Design review of the part built by this model. Coordinates are the model's own, in mm. Give positions to 0.01 mm unless a question says otherwise; leave off trailing zeros. Loops run counter-clockwise (first coordinate to the right, second up) from the corner with the lowest first, then second, coordinate; pieces in that order, holes last. Notation, with made-up numbers: M -14,1.25 L 21,1.25 A15 cw 21,15.25 Z; hole C 8.25,9 d4. An arc over 180 degrees is marked long. Use a Markdown table: item, result. Add a question column.
(1) Add section A-A, the plane y = 5. Give the boundary of the cut face in (x, z).
(2) For probe 1 along X at (y, z) = (5.5, 0.4); probe 2 along X at (y, z) = (2.75, 1.05); probe 3 along Y at (x, z) = (1.5, 0.6), list the stretches that pass through material, from the lowest coordinate up.
(3) Add section C-C, the plane z = 0.5. State how many separate pieces and enclosed holes the cut face has, then the cut area to 3 significant figures.
(4) Draft analysis for pull direction X (two halves, no side actions). For faces 1 (the face through (-2.356, 5, 1)), 2 (the face through (14.89, 3.13, 0.74)), 3 (the face through (9, 5, 0)), state which applies: pulls with the +X half, pulls with the -X half, needs draft (parallel to the pull), parting line crosses it, or undercut.
(5) Insertion check: pin 1 Ø3 at (x, y) = (16.64, 4.73) entering from +Z. The pin has a flat end and moves straight along its axis. Give the tip position at first contact, or say it passes through.
(6) Add section B-B, the plane x = 15.5. Give the boundary of the cut face in (y, z).
Autodesk Inventor part; units mm, degrees
ref_plane "YZ Plane" through (0, 0, 0) normal (1, 0, 0) x (0, 1, 0)
ref_plane "XZ Plane" through (0, 0, 0) normal (0, 1, 0) x (-1, 0, 0)
ref_plane "XY Plane" through (0, 0, 0) normal (0, 0, 1) x (1, 0, 0)
sketch "Sketch2" plane through (0, 0, 0) normal (0, 0, 1) x (1, 0, 0)
  circle A0 centre (1.6435, 4.7319) radius 2.125
  circle A1 centre (1.6435, 4.7319) radius 2.375
  line L0 (1.6435, 4.7319) -> (1.6435, 8.7319)
  line L1 (1.6435, 8.7319) -> (-2.3565, 8.7319)
  line L2 (-2.3565, 8.7319) -> (20.6435, 8.7319)
  line L3 (20.6435, 8.7319) -> (20.6435, 0.7319)
  line L4 (20.6435, 0.7319) -> (-2.3565, 0.7319)
  line L5 (-2.3565, 0.7319) -> (-2.3565, 8.7319)
  line L6 (9.1435, 8.7319) -> (9.1435, 2)
  circle A2 centre (16.6435, 4.7319) radius 2.375
  point P0 (0, 0)
  dimension "d0" = 4.75
  dimension "d1" = 4
  dimension "d2" = 4
  dimension "d3" = 23
  dimension "d4" = 8
extrude "Extrusion1" add sketch "Sketch2" along normal blind 1.5 contours L2 L3 L4 L5 L1
properties part number "Connector"
Established:
| question | item | result |
|---|---|---|
| 1 | outline | M -2.36,0 L -0.72,0 L -0.72,1.5 L -2.36,1.5 Z; M 4,0 L 14.28,0 L 14.28,1.5 L 4,1.5 Z; M 19,0 L 20.64,0 L 20.64,1.5 L 19,1.5 Z |
| 2 | probe 1 | -2.36 to -0.6, 3.89 to 14.4, 18.89 to 20.64 |
| 2 | probe 2 | -2.36 to 0.33, 2.95 to 15.33, 17.95 to 20.64 |
| 2 | probe 3 | 0.73 to 2.36, 7.1 to 8.73 |
| 3 | separate pieces | 1 |
| 3 | enclosed holes | 2 |
| 3 | area | 149 mm^2 |
| 4 | face 1 | pulls with the -X half |
| 4 | face 2 | undercut |
| 4 | face 3 | needs draft |
| 5 | pin 1 | through |
| 6 | outline | M 0.73,0 L 2.65,0 L 2.65,1.5 L 0.73,1.5 Z; M 6.81,0 L 8.73,0 L 8.73,1.5 L 6.81,1.5 Z |
